The model under review builds one solid part; all positions refer to its coordinate system, in mm. Round coordinates to 2 decimals unless told otherwise and drop trailing zeros. Order: outer loops, then holes, each group sorted by start corner. A loop starts at its lowest first (then second) coordinate and runs counter-clockwise, first axis right, second up. Notation, with made-up numbers: M -25,12 L 31,12 A25 ccw 31,49 Z; hole C 24.5,16 d6. An arc over 180 degrees is marked long. Answer as a JSON object with one key per item and string values. Group by question number.
1) Consider section B-B, the plane y = -1.25. Write out the cut boundary in (x, z).
2) Insertion check: pin 1 Ø5 at (x, y) = (2.5, 2) entering from -Z. The pin has a flat end and moves straight along its axis. Give the tip position at first contact, or say it passes through.
3) To check wall thickness, follow line 1 (X direction, y = -3.75, z = 0.1); line 2 (X direction, y = -5.5, z = 0.1); line 3 (X direction, y = 4.25, z = 0.15). State the ranges of each line that lie inside material, in increasing order.
4) Consider section A-A, the plane x = 0. Write out the cut boundary in (y, z), then the cut area to 3 significant figures.
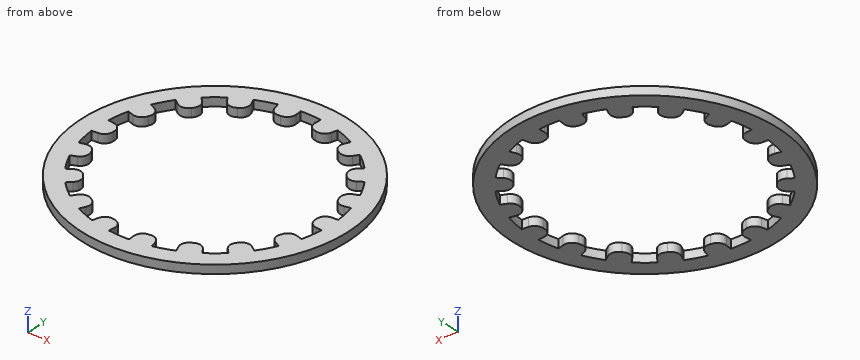
```python
from build123d import *

# Parameters (mm, degrees)
SKETCH1_R                = 7.8994
BOSS_EXTRUDE1_DEPTH      = 0.254
BOSS_EXTRUDE1_DEPTH_BACK = 0.254


with BuildPart() as part:
    # Sketch1 → Boss-Extrude1 (new body, two sides)
    with BuildSketch(Plane.XY) as boss_extrude1_sk:
        Circle(SKETCH1_R)
        with BuildLine():
            Line((-6.869858258, 0.601034718), (-6.508618542, 0.569430338))
            ThreePointArc((-6.508618542, 0.569430338), (-6.15764295, 0.382488604), (-6.048860848, 0))
            ThreePointArc((-6.048860848, 0), (-6.15764295, -0.382488604), (-6.508618542, -0.569430338))
            Line((-6.508618542, -0.569430338), (-6.869858258, -0.601034718))
            ThreePointArc((-6.869858258, -0.601034718), (-6.791332746, -1.197495198), (-6.661121091, -1.784842017))
            Line((-6.661121091, -1.784842017), (-6.310857462, -1.69098916))
            ThreePointArc((-6.310857462, -1.69098916), (-5.917110449, -1.746616205), (-5.684069903, -2.068832254))
            ThreePointArc((-5.684069903, -2.068832254), (-5.655472834, -2.465459643), (-5.92134417, -2.761168133))
            Line((-5.92134417, -2.761168133), (-6.24998913, -2.914417795))
            ThreePointArc((-6.24998913, -2.914417795), (-5.972197787, -3.44805), (-5.648954413, -3.955440463))
            Line((-5.648954413, -3.955440463), (-5.351913832, -3.747450409))
            ThreePointArc((-5.351913832, -3.747450409), (-4.9628871, -3.665053323), (-4.63369624, -3.888132806))
            ThreePointArc((-4.63369624, -3.888132806), (-4.471169229, -4.251059863), (-4.619868301, -4.619868301))
            Line((-4.619868301, -4.619868301), (-4.876279074, -4.876279074))
            ThreePointArc((-4.876279074, -4.876279074), (-4.432727635, -5.282719084), (-3.955440463, -5.648954413))
            Line((-3.955440463, -5.648954413), (-3.747450409, -5.351913832))
            ThreePointArc((-3.747450409, -5.351913832), (-3.410066323, -5.14143092), (-3.024430424, -5.238467158))
            ThreePointArc((-3.024430424, -5.238467158), (-2.747576627, -5.523919524), (-2.761168133, -5.92134417))
            Line((-2.761168133, -5.92134417), (-2.914417795, -6.24998913))
            ThreePointArc((-2.914417795, -6.24998913), (-2.35860511, -6.480214282), (-1.784842017, -6.661121091))
            Line((-1.784842017, -6.661121091), (-1.69098916, -6.310857462))
            ThreePointArc((-1.69098916, -6.310857462), (-1.44594122, -5.997676068), (-1.050373663, -5.95696506))
            ThreePointArc((-1.050373663, -5.95696506), (-0.692585734, -6.130512966), (-0.569430338, -6.508618542))
            Line((-0.569430338, -6.508618542), (-0.601034718, -6.869858258))
            ThreePointArc((-0.601034718, -6.869858258), (0, -6.8961), (0.601034718, -6.869858258))
            Line((0.601034718, -6.869858258), (0.569430338, -6.508618542))
            ThreePointArc((0.569430338, -6.508618542), (0.692585734, -6.130512966), (1.050373663, -5.95696506))
            ThreePointArc((1.050373663, -5.95696506), (1.44594122, -5.997676068), (1.69098916, -6.310857462))
            Line((1.69098916, -6.310857462), (1.784842017, -6.661121091))
            ThreePointArc((1.784842017, -6.661121091), (2.35860511, -6.480214282), (2.914417795, -6.24998913))
            Line((2.914417795, -6.24998913), (2.761168133, -5.92134417))
            ThreePointArc((2.761168133, -5.92134417), (2.747576627, -5.523919524), (3.024430424, -5.238467158))
            ThreePointArc((3.024430424, -5.238467158), (3.410066323, -5.14143092), (3.747450409, -5.351913832))
            Line((3.747450409, -5.351913832), (3.955440463, -5.648954413))
            ThreePointArc((3.955440463, -5.648954413), (4.432727635, -5.282719084), (4.876279074, -4.876279074))
            Line((4.876279074, -4.876279074), (4.619868301, -4.619868301))
            ThreePointArc((4.619868301, -4.619868301), (4.471169229, -4.251059863), (4.63369624, -3.888132806))
            ThreePointArc((4.63369624, -3.888132806), (4.9628871, -3.665053323), (5.351913832, -3.747450409))
            Line((5.351913832, -3.747450409), (5.648954413, -3.955440463))
            ThreePointArc((5.648954413, -3.955440463), (5.972197787, -3.44805), (6.24998913, -2.914417795))
            Line((6.24998913, -2.914417795), (5.92134417, -2.761168133))
            ThreePointArc((5.92134417, -2.761168133), (5.655472834, -2.465459643), (5.684069903, -2.068832254))
            ThreePointArc((5.684069903, -2.068832254), (5.917110449, -1.746616205), (6.310857462, -1.69098916))
            Line((6.310857462, -1.69098916), (6.661121091, -1.784842017))
            ThreePointArc((6.661121091, -1.784842017), (6.791332746, -1.197495198), (6.869858258, -0.601034718))
            Line((6.869858258, -0.601034718), (6.508618542, -0.569430338))
            ThreePointArc((6.508618542, -0.569430338), (6.15764295, -0.382488604), (6.048860848, 0))
            ThreePointArc((6.048860848, 0), (6.15764295, 0.382488604), (6.508618542, 0.569430338))
            Line((6.508618542, 0.569430338), (6.869858258, 0.601034718))
            ThreePointArc((6.869858258, 0.601034718), (6.791332746, 1.197495198), (6.661121091, 1.784842017))
            Line((6.661121091, 1.784842017), (6.310857462, 1.69098916))
            ThreePointArc((6.310857462, 1.69098916), (5.917110449, 1.746616205), (5.684069903, 2.068832254))
            ThreePointArc((5.684069903, 2.068832254), (5.655472834, 2.465459643), (5.92134417, 2.761168133))
            Line((5.92134417, 2.761168133), (6.24998913, 2.914417795))
            ThreePointArc((6.24998913, 2.914417795), (5.972197787, 3.44805), (5.648954413, 3.955440463))
            Line((5.648954413, 3.955440463), (5.351913832, 3.747450409))
            ThreePointArc((5.351913832, 3.747450409), (4.9628871, 3.665053323), (4.63369624, 3.888132806))
            ThreePointArc((4.63369624, 3.888132806), (4.471169229, 4.251059863), (4.619868301, 4.619868301))
            Line((4.619868301, 4.619868301), (4.876279074, 4.876279074))
            ThreePointArc((4.876279074, 4.876279074), (4.432727635, 5.282719084), (3.955440463, 5.648954413))
            Line((3.955440463, 5.648954413), (3.747450409, 5.351913832))
            ThreePointArc((3.747450409, 5.351913832), (3.410066323, 5.14143092), (3.024430424, 5.238467158))
            ThreePointArc((3.024430424, 5.238467158), (2.747576627, 5.523919524), (2.761168133, 5.92134417))
            Line((2.761168133, 5.92134417), (2.914417795, 6.24998913))
            ThreePointArc((2.914417795, 6.24998913), (2.35860511, 6.480214282), (1.784842017, 6.661121091))
            Line((1.784842017, 6.661121091), (1.69098916, 6.310857462))
            ThreePointArc((1.69098916, 6.310857462), (1.44594122, 5.997676068), (1.050373663, 5.95696506))
            ThreePointArc((1.050373663, 5.95696506), (0.692585734, 6.130512966), (0.569430338, 6.508618542))
            Line((0.569430338, 6.508618542), (0.601034718, 6.869858258))
            ThreePointArc((0.601034718, 6.869858258), (0, 6.8961), (-0.601034718, 6.869858258))
            Line((-0.601034718, 6.869858258), (-0.569430338, 6.508618542))
            ThreePointArc((-0.569430338, 6.508618542), (-0.692585734, 6.130512966), (-1.050373663, 5.95696506))
            ThreePointArc((-1.050373663, 5.95696506), (-1.44594122, 5.997676068), (-1.69098916, 6.310857462))
            Line((-1.69098916, 6.310857462), (-1.784842017, 6.661121091))
            ThreePointArc((-1.784842017, 6.661121091), (-2.35860511, 6.480214282), (-2.914417795, 6.24998913))
            Line((-2.914417795, 6.24998913), (-2.761168133, 5.92134417))
            ThreePointArc((-2.761168133, 5.92134417), (-2.747576627, 5.523919524), (-3.024430424, 5.238467158))
            ThreePointArc((-3.024430424, 5.238467158), (-3.410066323, 5.14143092), (-3.747450409, 5.351913832))
            Line((-3.747450409, 5.351913832), (-3.955440463, 5.648954413))
            ThreePointArc((-3.955440463, 5.648954413), (-4.432727635, 5.282719084), (-4.876279074, 4.876279074))
            Line((-4.876279074, 4.876279074), (-4.619868301, 4.619868301))
            ThreePointArc((-4.619868301, 4.619868301), (-4.471169229, 4.251059863), (-4.63369624, 3.888132806))
            ThreePointArc((-4.63369624, 3.888132806), (-4.9628871, 3.665053323), (-5.351913832, 3.747450409))
            Line((-5.351913832, 3.747450409), (-5.648954413, 3.955440463))
            ThreePointArc((-5.648954413, 3.955440463), (-5.972197787, 3.44805), (-6.24998913, 2.914417795))
            Line((-6.24998913, 2.914417795), (-5.92134417, 2.761168133))
            ThreePointArc((-5.92134417, 2.761168133), (-5.655472834, 2.465459643), (-5.684069903, 2.068832254))
            ThreePointArc((-5.684069903, 2.068832254), (-5.917110449, 1.746616205), (-6.310857462, 1.69098916))
            Line((-6.310857462, 1.69098916), (-6.661121091, 1.784842017))
            ThreePointArc((-6.661121091, 1.784842017), (-6.791332746, 1.197495198), (-6.869858258, 0.601034718))
        make_face(mode=Mode.SUBTRACT)
    extrude(amount=BOSS_EXTRUDE1_DEPTH)
    extrude(boss_extrude1_sk.sketch, amount=-BOSS_EXTRUDE1_DEPTH_BACK)


solid = part.part
```
Results list:
{
 "1": {"outline": "M -7.8,-0.25 L -6.78,-0.25 L -6.78,0.25 L -7.8,0.25 Z; M 6.78,-0.25 L 7.8,-0.25 L 7.8,0.25 L 6.78,0.25 Z"},
 "2": {"pin 1": "through"},
 "3": {"line 1": "-6.95 to -5.79, -5.36 to -4.77, 4.77 to 5.36, 5.79 to 6.95", "line 2": "-5.67 to -4.16, -3.85 to -2.76, 2.76 to 3.85, 4.16 to 5.67", "line 3": "-6.66 to -4.47, 4.47 to 6.66"},
 "4": {"outline": "M -7.9,-0.25 L -6.9,-0.25 L -6.9,0.25 L -7.9,0.25 Z; M 6.9,-0.25 L 7.9,-0.25 L 7.9,0.25 L 6.9,0.25 Z", "area": "1.02 mm^2"}
}
